Can you work these out from the drawing? Everything is in mm from the part's minimum corner. Give positions to 0.01 mm unless a question says otherwise; leave off trailing zeros. Order: outer loops, then holes, each group sorted by start corner. A loop starts at its lowest first (then second) coordinate and runs counter-clockwise, first axis right, second up. Notation, with made-up numbers: M 26,27 L 69,27 A38 cw 69,65 Z; hole C 14.25,-33 d3. An arc over 180 degrees is marked long. Answer as a JSON object with one key per item and string values.
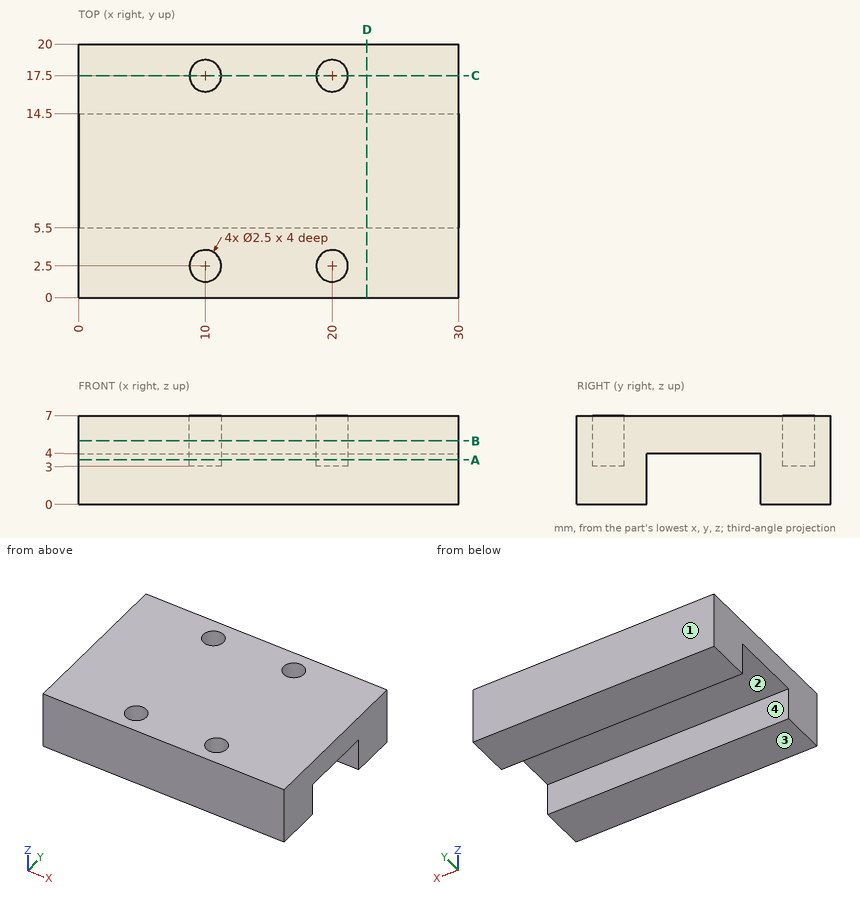
1) I want a section at D-D on x = 22.75. Write out the boundary of the cut face in (y, z), and give its area (3 significant figures).
Results found:
{"outline": "M 0,0 L 5.5,0 L 5.5,4 L 14.5,4 L 14.5,0 L 20,0 L 20,7 L 0,7 Z", "area": "104 mm²"}
2) I need wall thicknesses on L1, parallel to Y at x = 20, z = 6; L2, parallel to Y at x = 12.5, z = 3; L3, parallel to Z at x = 14.5, y = 11.5. Which ranges of each line are inside material? Lowest first, please.
Results found:
{"L1": "y = 0 to 1.25, 3.75 to 16.25, 18.75 to 20", "L2": "y = 0 to 5.5, 14.5 to 20", "L3": "z = 4 to 7"}
3) I want a section at B-B on z = 5. Write out the boundary of the cut face in (x, y).
Results found:
{"outline": "M 0,0 L 30,0 L 30,20 L 0,20 Z; hole C 10,2.5 d2.5; hole C 10,17.5 d2.5; hole C 20,2.5 d2.5; hole C 20,17.5 d2.5"}
4) I'm going to push flat-ended pins straight in: pin 1 Ø1 at (x, z) = (10.5, 2.5) entering from -Y; pin 2 Ø4.5 at (x, y) = (12, 8.5) entering from -Z; pin 3 Ø2 at (x, y) = (20, 17.5) entering from +Z. Where does each tip first touch, or does it pass through?
Results found:
{"pin 1": "stops at y = 0", "pin 2": "stops at z = 4", "pin 3": "stops at z = 3"}
5) I want a section at A-A on z = 3.5. Write out the boundary of the cut face in (x, y).
Results found:
{"outline": "M 0,0 L 30,0 L 30,5.5 L 0,5.5 Z; M 0,14.5 L 30,14.5 L 30,20 L 0,20 Z; hole C 10,2.5 d2.5; hole C 10,17.5 d2.5; hole C 20,2.5 d2.5; hole C 20,17.5 d2.5"}
6) I want a section at C-C on y = 17.5. Write out the boundary of the cut face in (x, z), and give its area (3 significant figures).
Results found:
{"outline": "M 0,0 L 30,0 L 30,7 L 21.25,7 L 21.25,3 L 18.75,3 L 18.75,7 L 11.25,7 L 11.25,3 L 8.75,3 L 8.75,7 L 0,7 Z", "area": "190 mm²"}
7) Thinking about a two-plate mould opening in Y: for the marked faces 1, 2, 3 and 4, which applies, pulls with the +Y half, pulls with the -Y half, needs draft (parallel to the pull), parting line crosses it, or undercut?
Results found:
{"face 1": "pulls with the +Y half", "face 2": "undercut", "face 3": "needs draft", "face 4": "undercut"}
